```python
from build123d import *

# Parameters (mm, degrees)
F2_W     = 10
F2_H     = 3
F3_DEPTH = 15
F4_R     = 4.99999
F5_R     = 2.5
F6_DEPTH = 18.6612540378
F7_W     = 2
F7_H     = 5
F7_W_2   = 5
F7_H_2   = 2
F8_DEPTH = 13.5


# Not quite as in the source:
# - a fillet or chamfer is up to 0.001 mm smaller than in the source, because OpenCascade refuses the exact size


with BuildPart() as f1:
    # F0 (on Top) → F1 (revolve)
    with BuildSketch(Plane.XY):
        Polygon((0, 6.2748147342), (-10, 6.2748147342), (-10, 1.304778154), (-5.5, 1.304778154), (-5.5, -14.7251852658), (-2.5, -14.7251852658), (-2.5, 1.2748147342), (0, 1.2748147342), align=None)
    revolve(axis=Axis((0, 3.7748147342, 0), (0, -1, 0)))

    # F2 (on face) → F3 (join)
    with BuildSketch(Plane(origin=(0, 6.2748147342, 0), x_dir=(-1, 0, 0), z_dir=(0, 1, 0))):
        with Locations((0, 7.1602540378)):
            Rectangle(F2_W, F2_H)
        with Locations((0, -7.1602540378)):
            Rectangle(F2_W, F2_H)
    extrude(amount=F3_DEPTH)

    # F4 (radius 5 in the source; OpenCascade refuses exactly that, so slightly less here)
    f4_edges = [f1.edges().sort_by_distance(p)[0] for p in [
        (-5, 21.274815, -7.160254),
        (5, 21.274815, -7.160254),
        (5, 21.274815, 7.160254),
        (-5, 21.274815, 7.160254),
    ]]
    fillet(f4_edges, radius=F4_R)

    # F5 (on face) → F6 (cut, through all)
    with BuildSketch(Plane(origin=(0, 0, -8.6602540378), x_dir=(1, 0, 0), z_dir=(0, 0, -1))):
        with Locations((0, -14.2748147342)):
            Circle(F5_R)
    extrude(amount=-F6_DEPTH, mode=Mode.SUBTRACT)

    # F7 (on face) → F8 (cut)
    with BuildSketch(Plane.XZ.offset(14.7251852658)):
        with Locations((0, 3.7191687186)):
            Rectangle(F7_W, F7_H)
        with Locations((-3.7191687186, 0)):
            Rectangle(F7_W_2, F7_H_2)
        with Locations((0, -3.7191687186)):
            Rectangle(F7_W, F7_H)
        with Locations((3.7191687186, 0)):
            Rectangle(F7_W_2, F7_H_2)
    extrude(amount=-F8_DEPTH, mode=Mode.SUBTRACT)


solid = f1.part
```
Could you check a few things on this model? Use its own coordinates, in mm. A direction names the side the tool comes from. Round coordinates to 2 decimals unless told otherwise and drop trailing zeros. Loops run counter-clockwise (first coordinate to the right, second up) from the corner with the lowest first, then second, coordinate; pieces in that order, holes last. Notation, with made-up numbers: M -4,58.25 L 26,58.25 A15 cw 26,70.25 Z; hole C 62,55.5 d6. An arc over 180 degrees is marked long. Put each result on its own line as item: value.
Q1. Imagine slicing it at A-A (y = -4.5). Write out the boundary of the cut face in (x, z), then the cut area to 3 significant figures.
Check result:
outline: M -5.41,-1 A5.5 ccw -1,-5.41 L -1,-2.29 A2.5 cw -2.29,-1 Z; M -5.41,1 L -2.29,1 A2.5 cw -1,2.29 L -1,5.41 A5.5 ccw Z; M 1,-5.41 A5.5 ccw 5.41,-1 L 2.29,-1 A2.5 cw 1,-2.29 Z; M 1,2.29 A2.5 cw 2.29,1 L 5.41,1 A5.5 ccw 1,5.41 Z
area: 51.1 mm2
Q2. For pin 1 (1.1 mm diameter, centred on x = -2, z = -9.5, fed in from +Y); pin 2 (1.6 mm diameter, centred on x = 4, y = -6, fed in from -Z); pin 3 (8 mm diameter, centred on x = 0.5, y = 16.5, fed in from +Z), each with a flat end and sliding along its axis, tell me the tip position at first contact or that it passes through.
Check result:
pin 1: y = 6.27
pin 2: z = -4.47
pin 3: z = 8.66
Q3. Imagine slicing it at C-C (x = -3.25). Write out the boundary of the cut face in (y, z), then the cut area to 3 significant figures.
Check result:
outline: M -14.73,-4.44 L 1.3,-4.44 L 1.3,-9.46 L 6.27,-9.46 L 6.27,-8.66 L 20.07,-8.66 L 20.07,-5.66 L 6.27,-5.66 L 6.27,5.66 L 20.07,5.66 L 20.07,8.66 L 6.27,8.66 L 6.27,9.46 L 1.3,9.46 L 1.3,4.44 L -14.73,4.44 L -14.73,1 L -1.23,1 L -1.23,-1 L -14.73,-1 Z
area: 292 mm2
Q4. Thinking about a two-plate mould opening in Z: for faces 4 (the face through (5, 11, -7)), 5 (the face through (-2, 12, 8.66)), 6 (the face through (0, 1.275, 0)), which applies, released by +Z, released by -Z, zero draft, split by the parting line, or undercut?
Check result:
face 4: zero draft
face 5: released by +Z
face 6: undercut
Q5. Imagine slicing it at D-D (z = 0). Write out the boundary of the cut face in (x, y), then the cut area to 3 significant figures.
Check result:
outline: M -10,1.3 L -5.5,1.3 L -5.5,-1.23 L -2.5,-1.23 L -2.5,1.27 L 2.5,1.27 L 2.5,-1.23 L 5.5,-1.23 L 5.5,1.3 L 10,1.3 L 10,6.27 L -10,6.27 Z
area: 115 mm2
Q6. Imagine slicing it at B-B (z = 5). Write out the boundary of the cut face in (x, y), then the cut area to 3 significant figures.
Check result:
outline: M -8.66,1.3 L -2.29,1.3 L -2.29,-14.73 L -1,-14.73 L -1,-1.23 L 1,-1.23 L 1,-14.73 L 2.29,-14.73 L 2.29,1.3 L 8.66,1.3 L 8.66,6.27 L -8.66,6.27 Z
area: 133 mm2
Q7. On a 3-axis mill with a long thin cutter (end or side, diameter ignored), from which of +Z, -Z, +X, -X, +Y, -Y can I reach the whole of each face in a straight line? I mean faces 1 (the face through (0, 6.275, 9)), 2 (the face through (4, -1.225, 0)), 3 (the face through (1, -8, 4)). Say none if no direction works.
Check result:
face 1: +Z, +X, -X, +Y
face 2: +X, -X, -Y
face 3: +Z, -Z, -Y
Q8. I need wall thicknesses on probe 1 along Y at (x, z) = (0, 6.7); probe 2 along Z at (x, y) = (-2.25, 10); probe 3 along Y at (x, z) = (-7.75, -6.25). Which ranges of each line are inside material? Lowest first, please.
Check result:
probe 1: 1.3 to 11.77, 16.77 to 21.27
probe 2: -8.66 to -5.66, 5.66 to 8.66
probe 3: 1.3 to 6.27
